Verification items for the finished model (mm, model axes). A direction names the side the tool comes from. Round coordinates to 2 decimals unless told otherwise and drop trailing zeros. Order: outer loops, then holes, each group sorted by start corner. A loop starts at its lowest first (then second) coordinate and runs counter-clockwise, first axis right, second up. Notation, with made-up numbers: (-16.75, 33.25) -> (-10.75, 33.25) arc R22 cw to (-10.75, 51.25) -> close; hole circle Ø4 at (23, 71). An arc over 180 degrees is marked (long way). Return JSON: item names as keys, results as strings. Group by question number.
1) Section check A-A on y = 0. Enter the section's corners in (x, z).
2) Scan line: L1, parallel to X at y = -1, z = 0.5. Record every from-to range of solid material in increasing order.
3) Draft check along Y on faces 1 (the flat face through (28, -6, 1)), 2 (the flat face through (0, 14.5, 1)), 3 (the flat face through (27.5, 0, 1)). Enter one of: pulls with the +Y half, pulls with the -Y half, needs draft (parallel to the pull), parting line crosses it, or undercut.
4) Tool access check on faces 4 (the flat face through (-19, 0, 1.2)), 5 (the flat face through (28, 7, 1)), 6 (the flat face through (27.5, 11, 1)), 7 (the flat face through (27.5, -11, 1)). Record the directions out of +Z, -Z, +X, -X, +Y, -Y that give a thin tool (end or side, any length) a straight path to the whole face; none if there is none.
5) Depth check by flat-ended pin: pin 1 (0.8 mm diameter, centred on y = 1.5, z = 0.5, fed in from +X). Enter the tip coordinate at first touch or a pass-through.
```python
from build123d import *

# Parameters (mm, degrees)
EXTRUDE_1_DEPTH     = 1.5
SKETCH_2_W          = 0.3
SKETCH_2_H          = 5
SKETCH_2_H_2        = 4.4
SKETCH_2_H_3        = 3.8
SKETCH_2_H_4        = 3.2
SKETCH_2_H_5        = 2.6
CUT_EXTRUDE_1_DEPTH = 0.3


with BuildPart() as part:
    # 草图1 → 凸台-拉伸1 (new body)
    with BuildSketch(Plane.XY):
        Polygon((27.5, 8), (28, 8), (28, 5), (27.5, 5), (27.5, -5), (28, -5), (28, -8), (27.5, -8), (27.5, -14.5), (-27.5, -14.5), (-27.5, 14.5), (27.5, 14.5), align=None)
    extrude(amount=EXTRUDE_1_DEPTH)

    # 草图2 → 切除-拉伸1 (cut)
    with BuildSketch(Plane.XY.offset(1.5)):
        with BuildLine():
            Line((-20, 3), (-20, -3))
            ThreePointArc((-20, -3), (-17, 0), (-20, 3))
        make_face()
        with Locations((-20.65, 0)):
            Rectangle(SKETCH_2_W, SKETCH_2_H)
        with Locations((-21.45, 0)):
            Rectangle(SKETCH_2_W, SKETCH_2_H_2)
        with Locations((-22.25, 0)):
            Rectangle(SKETCH_2_W, SKETCH_2_H_3)
        with Locations((-23.05, 0)):
            Rectangle(SKETCH_2_W, SKETCH_2_H_4)
        with Locations((-23.85, 0)):
            Rectangle(SKETCH_2_W, SKETCH_2_H_5)
    extrude(amount=-CUT_EXTRUDE_1_DEPTH, mode=Mode.SUBTRACT)


solid = part.part
```
Check result:
{
 "1": {"outline": "(-27.5, 0) -> (27.5, 0) -> (27.5, 1.5) -> (-17, 1.5) -> (-17, 1.2) -> (-20, 1.2) -> (-20, 1.5) -> (-20.5, 1.5) -> (-20.5, 1.2) -> (-20.8, 1.2) -> (-20.8, 1.5) -> (-21.3, 1.5) -> (-21.3, 1.2) -> (-21.6, 1.2) -> (-21.6, 1.5) -> (-22.1, 1.5) -> (-22.1, 1.2) -> (-22.4, 1.2) -> (-22.4, 1.5) -> (-22.9, 1.5) -> (-22.9, 1.2) -> (-23.2, 1.2) -> (-23.2, 1.5) -> (-23.7, 1.5) -> (-23.7, 1.2) -> (-24, 1.2) -> (-24, 1.5) -> (-27.5, 1.5) -> close"},
 "2": {"L1": "-27.5 to 27.5"},
 "3": {"face 1": "needs draft", "face 2": "pulls with the +Y half", "face 3": "undercut"},
 "4": {"face 4": "+Z", "face 5": "+Z, -Z, +X, +Y, -Y", "face 6": "+Z, -Z, +X, +Y", "face 7": "+Z, -Z, +X, -Y"},
 "5": {"pin 1": "x = 27.5"}
}
